The listing builds one solid part. Answer for the finished solid, in the listing's coordinates (mm). A direction names the side the tool comes from. Give positions to 0.01 mm unless a question says otherwise; leave off trailing zeros. Write each loop counter-clockwise with the first axis right and the second up, starting at its lowest first coordinate (ties: lowest second). Pieces come first, ordered by that corner, then holes. Notation, with made-up numbers: (17, 51) - (29, 51) arc R22 cw to (29, 89) - close; hole circle Ø10 at (80.5, 48.25). An arc over 180 degrees is marked (long way). Answer as CSV lines item,"result". Start each with the question number.
(1) This flat-tipped pin is pushed along its axis until it touches: pin 1 Ø13 at (x, y) = (40.55, -127) entering from -Z (3 decimals). Where does it stop, or does it pass through?
(2) Straight lines are drawn through the part: probe 1 along X at (y, z) = (132, 1.5); probe 2 along Y at (x, z) = (118, 0.75); probe 3 along Y at (x, z) = (3, 2.5). For each, find the intervals that lie inside material, in ascending order.
(3) Find section B-B (y = -127). Write down the section's boundary in (x, z) (3 decimals).
(4) Find section D-D (y = -37). Write down the section's boundary in (x, z) (3 decimals), then the cut area to 3 significant figures.
(5) Find section C-C (z = 0.25). State how many separate pieces and enclosed holes the cut face has, then the cut area to 3 significant figures.
(6) For faces 3 (the face through (-109.49, 57.4, 0.04)), 4 (the face through (-21.58, -16.32, -0.04)), determine the directions among +Z, -Z, +X, -X, +Y, -Y from which every point of the face is accessible in a straight line to the end or side of a thin tool.
(7) Find section A-A (y = 132.08). Write down the section's boundary in (x, z) (3 decimals), then the cut area to 3 significant figures.
(8) For a pull along Y with two mould halves and no side action, classify faces 1 (the face through (-2, 2, 3.175)), 2 (the face through (-30.33, 52.07, 0.04)) as pulls with the +Y half, pulls with the -Y half, needs draft (parallel to the pull), parting line crosses it, or undercut.
from build123d import *

# Parameters (mm, degrees)
F0_W      = 304.8
F0_H      = 304.8
F1_DEPTH  = 3.175
F2_W      = 177.8
F2_H      = 88.9
F3_DEPTH  = 6.351
F4_R      = 12.7
F5_R      = 5.75437
F6_DEPTH  = 6.351
F7_R      = 4.2164
F8_DEPTH  = 6.351
F9_R      = 4.2164
F10_DEPTH = 6.351
F11_R     = 3.175
F12_DEPTH = 6.351
F13_R     = 3.2639
F14_DEPTH = 6.351
F15_R     = 2.4892
F16_DEPTH = 25.4


with BuildPart() as f1:
    # F0 (on Top) → F1 (new body, symmetric)
    with BuildSketch(Plane.XY):
        Rectangle(F0_W, F0_H)
    extrude(amount=F1_DEPTH, both=True)

    # F2 (on face) → F3 (cut, through all)
    with BuildSketch(Plane.XY.offset(3.175)):
        with Locations((63.5, -57.15)):
            Rectangle(F2_W, F2_H)
    extrude(amount=-F3_DEPTH, mode=Mode.SUBTRACT)

    # F4
    f4_edges = [f1.edges().sort_by_distance(p)[0] for p in [
        (-25.4, -12.7, 0),
        (-25.4, -101.6, 0),
    ]]
    fillet(f4_edges, radius=F4_R)

    # F5 (on face) → F6 (cut, through all)
    with BuildSketch(Plane.XY.offset(3.175)):
        with Locations((40.55237, -127)):
            Circle(F5_R)
        with Locations((141.43863, -127)):
            Circle(F5_R)
        with Locations((40.55237, 12.7)):
            Circle(F5_R)
        with Locations((141.43863, 12.7)):
            Circle(F5_R)
    extrude(amount=-F6_DEPTH, mode=Mode.SUBTRACT)

    # F7 (on face) → F8 (cut, through all)
    with BuildSketch(Plane.XY.offset(3.175)):
        with Locations((-31.75, 132.08)):
            Circle(F7_R)
        with Locations((1.257298, 82.042)):
            Circle(F7_R)
    extrude(amount=-F8_DEPTH, mode=Mode.SUBTRACT)

    # F9 (on face) → F10 (cut, through all)
    with BuildSketch(Plane.XY.offset(3.175)):
        with Locations((-111.76, 53.848)):
            Circle(F9_R)
        with Locations((-34.349984, 50.8)):
            Circle(F9_R)
    extrude(amount=-F10_DEPTH, mode=Mode.SUBTRACT)

    # F11 (on face) → F12 (cut, through all)
    with BuildSketch(Plane.XY.offset(3.175)):
        with Locations((15.24, 102.616)):
            Circle(F11_R)
        with Locations((15.24, 39.116)):
            Circle(F11_R)
    extrude(amount=-F12_DEPTH, mode=Mode.SUBTRACT)

    # F13 (on face) → F14 (cut, through all)
    with BuildSketch(Plane.XY.offset(3.175)):
        with Locations((-48.4378, -98.806)):
            Circle(F13_R)
        with Locations((-128.7018, -61.468)):
            Circle(F13_R)
        with Locations((-117.729, -109.9312)):
            Circle(F13_R)
        with Locations((-37.4142, -61.468)):
            Circle(F13_R)
        with Locations((-48.4378, -15.494)):
            Circle(F13_R)
        with Locations((-117.729, -4.3688)):
            Circle(F13_R)
    extrude(amount=-F14_DEPTH, mode=Mode.SUBTRACT)

    # F15 (on face) → F16 (cut)
    with BuildSketch(Plane.XY.offset(3.175)):
        with Locations((-21.8948, 62.8904)):
            Circle(F15_R)
        with Locations((-33.782, 108.4072)):
            Circle(F15_R)
        with Locations((4.237579, 64.135)):
            Circle(F15_R)
    extrude(amount=-F16_DEPTH, mode=Mode.SUBTRACT)


solid = f1.part
Result set:
1,pin 1,"z = -3.175"
2,probe 1,"-152.4 to -35.97, -27.53 to 152.4"
2,probe 2,"-152.4 to -101.6, -12.7 to 152.4"
2,probe 3,"-152.4 to -101.6, -12.7 to 61.98, 66.29 to 78.2, 85.88 to 152.4"
3,outline,"(-152.4, -3.175) - (34.798, -3.175) - (34.798, 3.175) - (-152.4, 3.175) - close; (46.307, -3.175) - (135.684, -3.175) - (135.684, 3.175) - (46.307, 3.175) - close; (147.193, -3.175) - (152.4, -3.175) - (152.4, 3.175) - (147.193, 3.175) - close"
4,outline,"(-152.4, -3.175) - (-25.4, -3.175) - (-25.4, 3.175) - (-152.4, 3.175) - close"
4,area,"806 mm^2"
5,separate pieces,"1"
5,enclosed holes,"19"
5,area,"76,200 mm^2"
6,face 3,"+Z, -Z"
6,face 4,"+Z, -Z, +X"
7,outline,"(-152.4, -3.175) - (-35.966, -3.175) - (-35.966, 3.175) - (-152.4, 3.175) - close; (-27.534, -3.175) - (152.4, -3.175) - (152.4, 3.175) - (-27.534, 3.175) - close"
7,area,"1,880 mm^2"
8,face 1,"needs draft"
8,face 2,"undercut"
